```python
from build123d import *

# Parameters (mm, degrees)
SKETCH1_W           = 35.56
SKETCH1_H           = 10.16
SKETCH1_R           = 1.905
BOSS_EXTRUDE1_DEPTH = 5.08
SKETCH2_W           = 8.89
SKETCH2_H           = 2.54
CUT_EXTRUDE1_DEPTH  = 22.098824612
FILLET1_R           = 1.5875
FILLET2_R           = 0.635


with BuildPart() as part:
    # Sketch1 → Boss-Extrude1 (new body)
    with BuildSketch(Plane.XY):
        Rectangle(SKETCH1_W, SKETCH1_H)
        with Locations((-12.7, 0)):
            Circle(SKETCH1_R, mode=Mode.SUBTRACT)
        with Locations((12.7, 0)):
            Circle(SKETCH1_R, mode=Mode.SUBTRACT)
    extrude(amount=BOSS_EXTRUDE1_DEPTH)

    # Sketch2 → Cut-Extrude1 (cut, through all)
    with BuildSketch(Plane.XZ.offset(5.08)):
        Polygon((0, 0), (-5.715, 0), (-5.715, 3.175), (1.905, 3.175), (1.905, 1.27), (5.715, 1.27), (5.715, 0), align=None)
        with Locations((-13.335, 3.81)):
            Rectangle(SKETCH2_W, SKETCH2_H)
        with Locations((13.335, 3.81)):
            Rectangle(SKETCH2_W, SKETCH2_H)
    extrude(amount=-CUT_EXTRUDE1_DEPTH, mode=Mode.SUBTRACT)

    # Fillet1
    fillet1_edges = [part.edges().sort_by_distance(p)[0] for p in [
        (-17.78, 0, 2.54),
        (-8.89, 0, 5.08),
        (8.89, 0, 5.08),
        (17.78, 0, 2.54),
    ]]
    fillet(fillet1_edges, radius=FILLET1_R)

    # Fillet2
    fillet2_edges = [part.edges().sort_by_distance(p)[0] for p in [
        (-5.715, 0, 3.175),
        (1.905, 0, 3.175),
        (1.905, 0, 1.27),
        (5.715, 0, 1.27),
    ]]
    fillet(fillet2_edges, radius=FILLET2_R)


solid = part.part
```
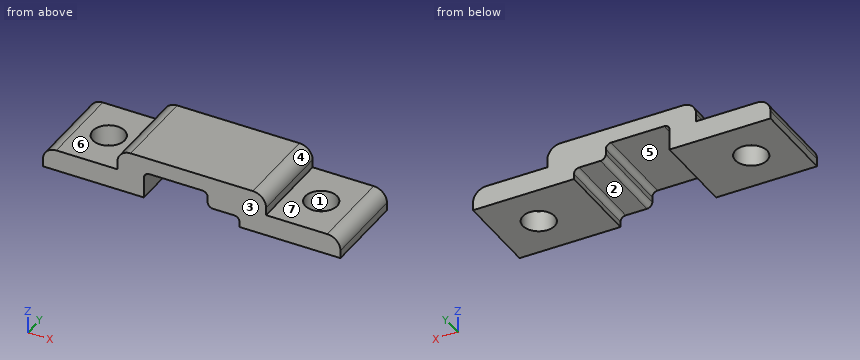
Here's how the part is built. I have some questions about the finished solid (model axes, mm). Face numbers are marked on the shaded views. A direction names the side the tool comes from. Round coordinates to 2 decimals unless told otherwise and drop trailing zeros. Loops run counter-clockwise (first coordinate to the right, second up) from the corner with the lowest first, then second, coordinate; pieces in that order, holes last.
1. Suppose I cut it at D-D, the plane x = 14. Please give me the cut outline in (y, z).
Answers:
outline: (-5.08, 0) - (-1.39, 0) - (-1.39, 2.54) - (-5.08, 2.54) - close; (1.39, 0) - (5.08, 0) - (5.08, 2.54) - (1.39, 2.54) - close
2. Will these pins go through, and if not, where does the flat tip stop? pin 1 (3 mm diameter, centred on x = -2, y = 2, fed in from -Z) (3 decimals); pin 2 (0.8 mm diameter, centred on y = -1.5, z = 3, fed in from -X); pin 3 (2 mm diameter, centred on x = 12, y = -1, fed in from +Z).
Answers:
pin 1: stops at z = 3.175
pin 2: stops at x = -8.89
pin 3: stops at z = 2.54
3. Thinking about a two-plate mould opening in X: for the marked faces 1, 2, 3 and 4, which applies, released by +X, released by -X, zero draft, split by the parting line, or undercut?
Answers:
face 1: undercut
face 2: undercut
face 3: zero draft
face 4: released by +X
4. For the marked faces 5, 6 and 7, which set-ups out of +Z, -Z, +X, -X, +Y, -Y let a thin tool reach every point of the face, with its end or its side?
Answers:
face 5: -Z, +Y, -Y
face 6: +Z, -X, +Y, -Y
face 7: +Z, +X, +Y, -Y
5. Suppose I cut it at A-A, the plane x = -12.7. Please give me the cut outline in (y, z) (3 decimals).
Answers:
outline: (-5.08, 0) - (-1.905, 0) - (-1.905, 2.54) - (-5.08, 2.54) - close; (1.905, 0) - (5.08, 0) - (5.08, 2.54) - (1.905, 2.54) - close
6. If I drill on probe 1 along Y at (x, z) = (-12.7, 1.4) (3 decimals); probe 2 along X at (y, z) = (0, 1.15) (3 decimals); probe 3 along X at (y, z) = (1.5, 1.2) (3 decimals), over which ranges is the centre line in solid material (lowest first)?
Answers:
probe 1: y = -5.08 to -1.905, 1.905 to 5.08
probe 2: x = -17.768 to -14.605, -10.795 to -5.715, 5.451 to 10.795, 14.605 to 17.768
probe 3: x = -17.761 to -13.874, -11.526 to -5.715, 5.37 to 11.526, 13.874 to 17.761
7. Suppose I cut it at C-C, the plane y = -2.25. Please give me the cut outline in (x, z) (1 decimal).
Answers:
outline: (-17.8, 0) - (-5.7, 0) - (-5.7, 2.5) arc R0.6 cw to (-5.1, 3.2) - (1.3, 3.2) arc R0.6 cw to (1.9, 2.5) - (1.9, 1.9) arc R0.6 ccw to (2.5, 1.3) - (5.1, 1.3) arc R0.6 cw to (5.7, 0.6) - (5.7, 0) - (17.8, 0) - (17.8, 1) arc R1.6 ccw to (16.2, 2.5) - (8.9, 2.5) - (8.9, 3.5) arc R1.6 ccw to (7.3, 5.1) - (-7.3, 5.1) arc R1.6 ccw to (-8.9, 3.5) - (-8.9, 2.5) - (-16.2, 2.5) arc R1.6 ccw to (-17.8, 1) - close
8. Suppose I cut it at B-B, the plane y = 0. Give the number of separate pieces and of enclosed holes in the cut face, and give its area (3 significant figures).
Answers:
separate pieces: 3
enclosed holes: 0
area: 85.1 mm2
